```python
from build123d import *

# Parameters (mm, degrees)
F1_DEPTH = 152.4
F2_DEPTH = 101.6
F3_R     = 14.611246
F4_DEPTH = 161.29


with BuildPart() as f1:
    # F0 (on Front) → F1 (new body, symmetric)
    with BuildSketch(Plane.XZ):
        with BuildLine():
            Line((67.64774, 0), (46.662122, 0))
            ThreePointArc((46.662122, 0), (0, -44.853662), (-46.662122, 0))
            Line((-46.662122, 0), (-67.64774, 0))
            ThreePointArc((-67.64774, 0), (0, -67.278411), (67.64774, 0))
        make_face()
    extrude(amount=F1_DEPTH, both=True)

    # F0 (on Front) → F2 (join, symmetric)
    with BuildSketch(Plane.XZ):
        with BuildLine():
            Line((93.324244, 0), (67.64774, 0))
            ThreePointArc((67.64774, 0), (0, -67.278411), (-67.64774, 0))
            Line((-67.64774, 0), (-93.324244, 0))
            Line((-93.324244, 0), (-93.324244, -118.506968))
            Line((-93.324244, -118.506968), (0, -118.506968))
            Line((0, -118.506968), (93.324244, -118.506968))
            Line((93.324244, -118.506968), (93.324244, 0))
        make_face()
    extrude(amount=F2_DEPTH, both=True)

    # F3 (on Top) → F4 (cut)
    with BuildSketch(Plane.XY):
        with Locations((-70.525467, 0)):
            Circle(F3_R)
        with Locations((70.525467, 0)):
            Circle(F3_R)
    extrude(amount=-F4_DEPTH, mode=Mode.SUBTRACT)


solid = f1.part
```
Check sheet for the modelled part. Datum: model origin and axes. Units: mm. A direction names the side the tool comes from. Round coordinates to 2 decimals unless told otherwise and drop trailing zeros. Write each loop counter-clockwise with the first axis right and the second up, starting at its lowest first coordinate (ties: lowest second). Pieces come first, ordered by that corner, then holes. Notation, with made-up numbers: (-39, -15.75) -> (-33, -15.75) arc R21 ccw to (-33, 7.25) -> close; hole circle Ø7 at (79.25, 88). An arc over 180 degrees is marked (long way). One line per question, with ' | ' between items. Start each with the question number.
1. Release check for a two-part mould opening along X. For faces 1 (the face through (-57.03, -5.6, -58.42)), 2 (the face through (-1, -152.4, -48)), 3 (the face through (-93.324, -1, -58)) record: +X half, -X half, draft (parallel to the pull), parting line (faces both ways), or undercut.
2. Set-up check for faces 4 (the face through (1.001, -2.134, -44.843)), 5 (the face through (-1.482, -127.356, -67.262)), 6 (the face through (-1.482, 126.644, -67.262)): record each of +Z, -Z, +X, -X, +Y, -Y from which the full face is reachable in a straight line by a thin tool's end or side.
3. Sectioned sample at C-C, the plane x = 0. Record the cut outline in (y, z).
4. Scan lines: line 1 along Y through (x, z) = (71.5, -53); line 2 along X through (y, z) = (8, -110.5); line 3 along Y through (x, z) = (-59, -109). Record each from-to range of solid material in increasing order. Write a range as from..to.
5. Sectioned sample at D-D, the plane z = -72.5. Record the cut outline in (x, y), then the cut area to 3 significant figures.
6. Sectioned sample at B-B, the plane z = -34. Record the cut outline in (x, y).
7. Depth check by flat-ended pin: pin 1 (12 mm diameter, centred on x = -49, z = -71.5, fed in from +Y); pin 2 (10 mm diameter, centred on x = -9.5, y = 5.5, fed in from +Z). Enter the tip coordinate at first touch or a pass-through.
8. Sectioned sample at A-A, the plane y = 0. Record the cut outline in (x, z).
Taken from the geometry:
1) face 1: undercut | face 2: draft | face 3: -X half
2) face 4: +Z, +Y, -Y | face 5: -Z, -Y | face 6: -Z, +Y
3) outline: (-152.4, -67.28) -> (-101.6, -67.28) -> (-101.6, -118.51) -> (101.6, -118.51) -> (101.6, -67.28) -> (152.4, -67.28) -> (152.4, -44.85) -> (-152.4, -44.85) -> close
4) line 1: y = -101.6..-14.58, 14.58..101.6 | line 2: x = -93.32..-82.75, -58.3..58.3, 82.75..93.32 | line 3: y = -101.6..-8.98, 8.98..101.6
5) outline: (-93.32, -101.6) -> (93.32, -101.6) -> (93.32, 101.6) -> (-93.32, 101.6) -> close; hole circle Ø29.22 at (-70.53, 0); hole circle Ø29.22 at (70.53, 0) | area: 36,600 mm^2
6) outline: (-93.32, -101.6) -> (-58.27, -101.6) -> (-58.27, -152.4) -> (-29.93, -152.4) -> (-29.93, 152.4) -> (-58.27, 152.4) -> (-58.27, 101.6) -> (-93.32, 101.6) -> close; (29.93, -152.4) -> (58.27, -152.4) -> (58.27, -101.6) -> (93.32, -101.6) -> (93.32, 101.6) -> (58.27, 101.6) -> (58.27, 152.4) -> (29.93, 152.4) -> close; hole circle Ø29.22 at (-70.53, 0); hole circle Ø29.22 at (70.53, 0)
7) pin 1: stops at y = 101.6 | pin 2: stops at z = -42.55
8) outline: (-93.32, -118.51) -> (-85.14, -118.51) -> (-85.14, 0) -> (-93.32, 0) -> close; (-55.91, -118.51) -> (55.91, -118.51) -> (55.91, 0) -> (46.66, 0) arc R46.7 cw to (-46.66, 0) -> (-55.91, 0) -> close; (85.14, -118.51) -> (93.32, -118.51) -> (93.32, 0) -> (85.14, 0) -> close
